CAD build for the part. Positions are in the model's coordinates, mm. A direction names the side the tool comes from. Round coordinates to 2 decimals unless told otherwise and drop trailing zeros. Write each loop counter-clockwise with the first axis right and the second up, starting at its lowest first coordinate (ties: lowest second). Pieces come first, ordered by that corner, then holes. Notation, with made-up numbers: (81.25, -28.75) - (111.25, -28.75) arc R12 cw to (111.25, -11.75) - close; hole circle Ø11 at (-28, 51). An arc over 180 degrees is marked (long way). Answer in a Markdown table with one row per item.
```python
from build123d import *

# Parameters (mm, degrees)
SKETCH_1_W          = 220
SKETCH_1_H          = 34
EXTRUDE_1_DEPTH     = 3
SKETCH_2_R          = 1.6
CUT_EXTRUDE_1_DEPTH = 5
SKETCH_3_R          = 1.6
CUT_EXTRUDE_3_DEPTH = 5
CUT_EXTRUDE_4_DEPTH = 5
FILLET_1_R          = 1


with BuildPart() as part:
    # 草图1 → 凸台-拉伸1 (new body)
    with BuildSketch(Plane.XY):
        Rectangle(SKETCH_1_W, SKETCH_1_H)
    extrude(amount=EXTRUDE_1_DEPTH)

    # 草图2 → 切除-拉伸1 (cut, symmetric)
    with BuildSketch(Plane.XY.offset(3)):
        with Locations(Location((-12.07, 13, 0), (0, 0, 180))):
            Circle(SKETCH_2_R)
        with Locations(Location((12.07, 13, 0), (0, 0, 180))):
            Circle(SKETCH_2_R)
        with Locations(Location((12.07, -13, 0), (0, 0, 180))):
            Circle(SKETCH_2_R)
        with Locations(Location((-12.07, -13, 0), (0, 0, 180))):
            Circle(SKETCH_2_R)
    extrude(amount=CUT_EXTRUDE_1_DEPTH, both=True, mode=Mode.SUBTRACT)

    # 草图3 → 切除-拉伸3 (cut, symmetric)
    with BuildSketch(Plane.XY.offset(3)):
        with BuildLine():
            ThreePointArc((-110, 10), (-108.873217569, 12.782915881), (-106.127689601, 13.997961401))
            Line((-106.127689601, 13.997961401), (-12.197689601, 16.997961401))
            ThreePointArc((-12.197689601, 16.997961401), (-12.133852914, 16.999490318), (-12.069999956, 17))
            Line((-12.069999956, 17), (-110, 17))
            Line((-110, 17), (-110, 10))
        make_face()
        with BuildLine():
            ThreePointArc((-106.127689601, -13.997961401), (-108.873217569, -12.782915881), (-110, -10))
            Line((-110, -10), (-110, -17))
            Line((-110, -17), (-12.070000078, -17))
            ThreePointArc((-12.070000078, -17), (-12.133852976, -16.999490317), (-12.197689601, -16.997961401))
            Line((-12.197689601, -16.997961401), (-106.127689601, -13.997961401))
        make_face()
        with Locations(Location((-106, -10, 0), (0, 0, 180))):
            Circle(SKETCH_3_R)
        with Locations(Location((-106, 10, 0), (0, 0, 180))):
            Circle(SKETCH_3_R)
    cut_extrude_3 = extrude(amount=CUT_EXTRUDE_3_DEPTH, both=True, mode=Mode.SUBTRACT)

    # 镜向1: 切除-拉伸3 across plane
    add(cut_extrude_3.mirror(Plane(origin=(0, 0, 0), x_dir=(0, 0, 1), z_dir=(1, 0, 0))), mode=Mode.SUBTRACT)

    # 草图4 → 切除-拉伸4 (cut, symmetric)
    with BuildSketch(Plane.XY.offset(3)):
        Polygon((-16.07, -11.319443342), (-16.07, 11.319443342), (-58.360424625, 0), align=None)
        Polygon((-64.161827726, 1.552801947), (-22.657455715, 12.661850664), (-96.817055288, 10.293291112), align=None)
        Polygon((-102, -8.574952764), (-69.963230826, 0), (-102, 8.574952764), align=None)
        Polygon((-22.657455715, -12.661850664), (-64.161827726, -1.552801947), (-96.817055288, -10.293291112), align=None)
        Polygon((-10.07, 6.988222073), (-10.07, -6.988222073), (-2.25095597, 0), align=None)
        Polygon((-7.81904403, 9), (0, 2.011777927), (7.81904403, 9), align=None)
        Polygon((10.07, 6.988222073), (2.25095597, 0), (10.07, -6.988222073), align=None)
        Polygon((0, -2.011777927), (-7.81904403, -9), (7.81904403, -9), align=None)
        Polygon((16.07, -11.319443342), (58.360424625, 0), (16.07, 11.319443342), align=None)
        Polygon((64.161827726, 1.552801947), (96.817055288, 10.293291112), (22.657455715, 12.661850664), align=None)
        Polygon((102, 8.574952764), (69.963230826, 0), (102, -8.574952764), align=None)
        Polygon((96.817055288, -10.293291112), (64.161827726, -1.552801947), (22.657455715, -12.661850664), align=None)
    extrude(amount=CUT_EXTRUDE_4_DEPTH, both=True, mode=Mode.SUBTRACT)

    # 圆角1
    fillet_1_edges = [part.edges().sort_by_distance(p)[0] for p in [
        (2.25095597, 0, 1.5),
        (10.07, 6.988222073, 1.5),
        (10.07, -6.988222073, 1.5),
        (0, 2.011777927, 1.5),
        (-7.81904403, 9, 1.5),
        (7.81904403, 9, 1.5),
        (-7.81904403, -9, 1.5),
        (0, -2.011777927, 1.5),
        (7.81904403, -9, 1.5),
        (16.07, 11.319443342, 1.5),
        (58.360424625, 0, 1.5),
        (16.07, -11.319443342, 1.5),
        (-102, -8.574952764, 1.5),
        (-102, 8.574952764, 1.5),
        (-69.963230826, 0, 1.5),
        (-96.817055288, 10.293291112, 1.5),
        (-22.657455715, 12.661850664, 1.5),
        (-64.161827726, 1.552801947, 1.5),
        (-64.161827726, -1.552801947, 1.5),
        (-22.657455715, -12.661850664, 1.5),
        (-96.817055288, -10.293291112, 1.5),
        (-10.07, -6.988222073, 1.5),
        (-10.07, 6.988222073, 1.5),
        (-2.25095597, 0, 1.5),
        (96.817055288, -10.293291112, 1.5),
        (22.657455715, -12.661850664, 1.5),
        (64.161827726, -1.552801947, 1.5),
        (22.657455715, 12.661850664, 1.5),
        (96.817055288, 10.293291112, 1.5),
        (64.161827726, 1.552801947, 1.5),
        (102, 8.574952764, 1.5),
        (102, -8.574952764, 1.5),
        (69.963230826, 0, 1.5),
        (-58.360424625, 0, 1.5),
        (-16.07, 11.319443342, 1.5),
        (-16.07, -11.319443342, 1.5),
    ]]
    fillet(fillet_1_edges, radius=FILLET_1_R)


solid = part.part
```
Q1. Flat gauge pins, fed straight in: pin 1 (1.9 mm diameter, centred on x = -106, y = -10, fed in from -Z); pin 2 (1.5 mm diameter, centred on x = -18.5, z = 0.5, fed in from +Y); pin 3 (1.5 mm diameter, centred on y = -11, z = 2, fed in from -X). Where does each tip first touch, or does it go through?
Computed:
| item | result |
|---|---|
| pin 1 | passes through |
| pin 2 | stops at y = 16.82 |
| pin 3 | stops at x = -109.99 |
Q2. Drill centre lines: line 1 (Y direction, x = -106, z = 1.5); line 2 (Y direction, x = -74, z = 0.9); line 3 (Y direction, x = -68.5, z = 1.1). Where is each one in solid material? Low to high.
Computed:
| item | result |
|---|---|
| line 1 | y = -14 to -11.6, -8.4 to 8.4, 11.6 to 14 |
| line 2 | y = -15.02 to -11.02, -4.19 to -1.08, 1.08 to 4.19, 11.02 to 15.02 |
| line 3 | y = -15.2 to -11.2, -2.71 to 2.71, 11.2 to 15.2 |
Q3. Saw through at A-A on x = 44.5. List the corners of the cut face in (y, z).
Computed:
| item | result |
|---|---|
| outline | (-15.97, 0) - (-11.96, 0) - (-11.96, 3) - (-15.97, 3) - close; (-6.82, 0) - (-3.71, 0) - (-3.71, 3) - (-6.82, 3) - close; (3.71, 0) - (6.82, 0) - (6.82, 3) - (3.71, 3) - close; (11.96, 0) - (15.97, 0) - (15.97, 3) - (11.96, 3) - close |
Q4. Saw through at B-B on z = 1.1. Count the separate pieces of the cut face and the enclosed holes in it, then the cut area to 3 significant figures.
Computed:
| item | result |
|---|---|
| separate pieces | 1 |
| enclosed holes | 20 |
| area | 3,690 mm2 |
Q5. Pull direction X, two halves, no side cores. Call faces 1 (the cylindrical face through (-108.843, -12.814, 1.479)), 2 (the flat face through (-2, 0, 3)), 3 (the flat face through (87.347, 4.653, 1.479)): released by +X, released by -X, zero draft, split by the parting line, or undercut.
Computed:
| item | result |
|---|---|
| face 1 | released by -X |
| face 2 | zero draft |
| face 3 | undercut |
Q6. 3-axis set-ups, long thin cutter, end or side, ignore diameter. For faces 4 (the flat face through (-2, 0, 0)), 5 (the flat face through (86.97, -4.55, 1.48)): which of +Z, -Z, +X, -X, +Y, -Y reach the whole face in a straight line?
Computed:
| item | result |
|---|---|
| face 4 | -Z, +X, -X, +Y, -Y |
| face 5 | +Z, -Z |
